Source: CAD feature listing. Evaluate the final solid. Frame: model axes, mm. A direction names the side the tool comes from. Round coordinates to 2 decimals unless told otherwise and drop trailing zeros. Write each loop counter-clockwise with the first axis right and the second up, starting at its lowest first coordinate (ties: lowest second). Pieces come first, ordered by that corner, then holes. Notation, with made-up numbers: (15, 55) - (58, 55) arc R22 cw to (58, 78) - close; hole circle Ø4 at (58, -18). An arc over 180 degrees is marked (long way). Write item = value, one per line. Start each with the question number.
```python
from build123d import *

# Parameters (mm, degrees)
CROQUIS1_R              = 2
CROQUIS1_W              = 19.8
CROQUIS1_H              = 2.8
SALIENTE_EXTRUIR1_DEPTH = 3


with BuildPart() as part:
    # Croquis1 → Saliente-Extruir1 (new body)
    with BuildSketch(Plane.XY):
        with BuildLine():
            Line((-40, 29), (40, 29))
            Line((40, 29), (40, -29))
            ThreePointArc((40, -29), (32.091883092, -48.091883092), (13, -56))
            Line((13, -56), (13, -68))
            Line((13, -68), (-10, -68))
            Line((-10, -68), (-10, -56))
            Line((-10, -56), (-40, -56))
            Line((-40, -56), (-40, 29))
        make_face()
        with Locations((1.5, -57.5)):
            Circle(CROQUIS1_R, mode=Mode.SUBTRACT)
        with Locations((0, -51.6)):
            Rectangle(CROQUIS1_W, CROQUIS1_H, mode=Mode.SUBTRACT)
    extrude(amount=SALIENTE_EXTRUIR1_DEPTH)


solid = part.part
```
(1) Section B-B (x = 1.5). Return the cut outline in (y, z), plus the area to 3 significant figures.
(2) Pull-direction query (Y, two-part tool) for faces 1 (the cylindrical face through (1.24, -55.517, 1.479)), 2 (the flat face through (-1, 29, 1)), 3 (the flat face through (40, 0, 1)); classes: +Y half, -Y half, draft (parallel to the pull), parting line (faces both ways), or undercut.
(3) Reachability of faces 4 (the flat face through (-10, -62, 1)), 5 (the flat face through (0, -50.2, 1)), 6 (the flat face through (13, -62, 1)) from +Z, -Z, +X, -X, +Y, -Y: full face, straight path, thin tool, end or side. Return the list, or none.
(4) Contact query for flat-ended pins moving along their axis: P1, Ø1.5, axis at x = -23, z = 2, coming from the -Y side; P2, Ø1.5, axis at y = -61.5, z = 2, coming from the +X side; P3, Ø3.5, axis at x = 1.5, y = -57.5, coming from the +Z side. Output: stop coordinate, or through.
(5) Section C-C (z = 2.25). Return the cut outline in (x, y).
(6) Section A-A (y = -57.5). Return the cut outline in (x, z).
(7) Ray query, L1, parallel to Y at x = 1.5, z = 1.35; L2, parallel to Y at x = -3, z = 2.3; L3, parallel to Y at x = -20, z = 0.75. Return the intervals inside material, ascending. Write a range as from..to.
(8) Section D-D (x = 29). Return the cut outline in (y, z), plus the area to 3 significant figures.
Solution:
q1.outline = (-68, 0) - (-59.5, 0) - (-59.5, 3) - (-68, 3) - close; (-55.5, 0) - (-53, 0) - (-53, 3) - (-55.5, 3) - close; (-50.2, 0) - (29, 0) - (29, 3) - (-50.2, 3) - close
q1.area = 271 mm^2
q2.face_1 = undercut
q2.face_2 = +Y half
q2.face_3 = draft
q3.face_4 = +Z, -Z, -X, -Y
q3.face_5 = +Z, -Z
q3.face_6 = +Z, -Z, +X, -Y
q4.P1 = -56
q4.P2 = 13
q4.P3 = through
q5.outline = (-40, -56) - (-10, -56) - (-10, -68) - (13, -68) - (13, -56) arc R27 ccw to (40, -29) - (40, 29) - (-40, 29) - close; hole (-9.9, -53) - (9.9, -53) - (9.9, -50.2) - (-9.9, -50.2) - close; hole circle Ø4 at (1.5, -57.5)
q6.outline = (-10, 0) - (-0.5, 0) - (-0.5, 3) - (-10, 3) - close; (3.5, 0) - (13, 0) - (13, 3) - (3.5, 3) - close
q7.L1 = -68..-59.5, -55.5..-53, -50.2..29
q7.L2 = -68..-53, -50.2..29
q7.L3 = -56..29
q8.outline = (-50.75, 0) - (29, 0) - (29, 3) - (-50.75, 3) - close
q8.area = 239 mm^2
